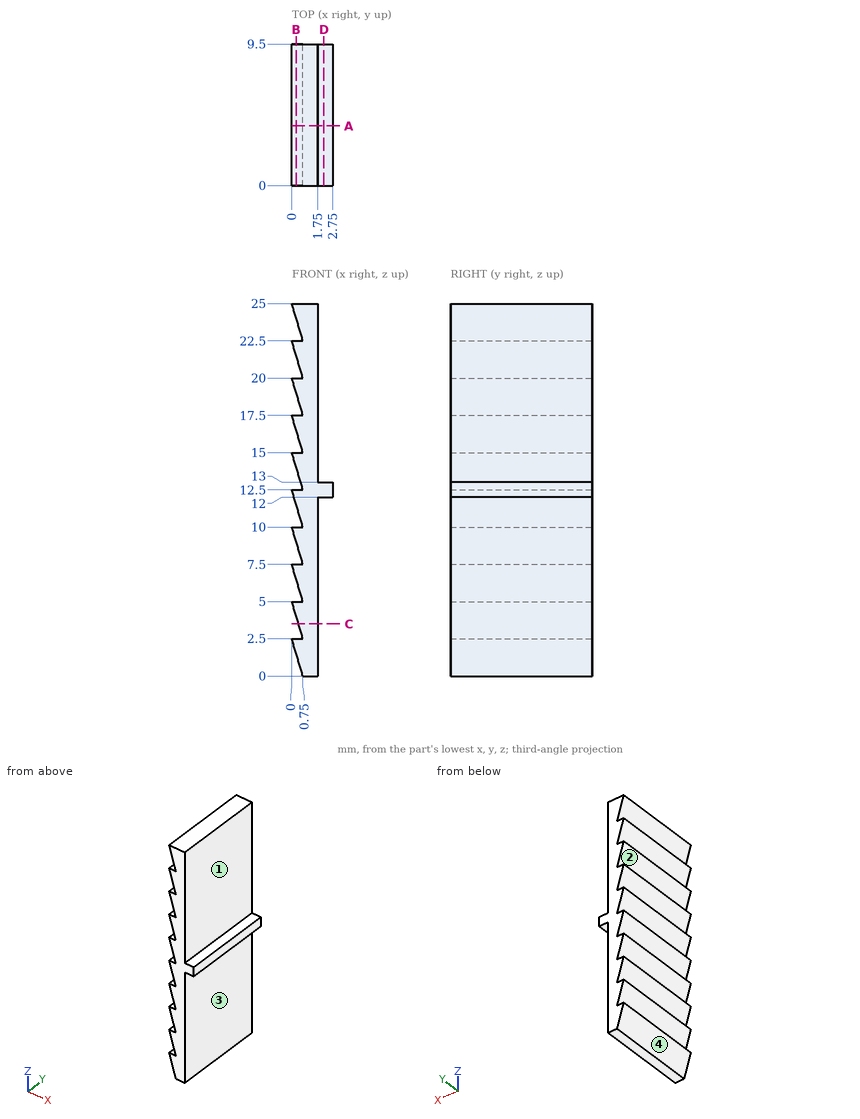
Geometry: see drawing. Coordinates: mm, zero at the bounding-box minimum. A direction names the side the tool comes from. Round coordinates to 2 decimals unless told otherwise and drop trailing zeros. Loops run counter-clockwise (first coordinate to the right, second up) from the corner with the lowest first, then second, coordinate; pieces in that order, holes last. Notation, with made-up numbers: (75, -30.5) -> (131, -30.5) arc R23 cw to (131, -3.5) -> close; hole circle Ø2 at (83, 83). An arc over 180 degrees is marked (long way). One line per question, with ' | ' between items. Start each with the question number.
1. Section B-B on x = 0.3. Count the separate pieces of the cut face and the enclosed holes in it, and give its area (3 significant figures).
2. Section D-D on x = 2.15. Output: boundary loops of the cut face in (y, z).
3. Set-up query: the marked faces 1, 2, 3 and 4. Return all of +Z, -Z, +X, -X, +Y, -Y with unobstructed straight access to the full face (end or side cutting, diameter ignored); none if empty.
4. Line query: line 1 along Z through (x, y) = (2.25, 1.25); line 2 along X through (y, z) = (9, 11.75) (3 decimals); line 3 along X through (y, z) = (0.75, 1.5). Output: solid intervals per line, ascending. Write a range as [from, to].
5. Section C-C on z = 3.5. Output: boundary loops of the cut face in (x, y), and give its area (4 significant figures).
6. Contact query for flat-ended pins moving along their axis: pin 1 (0.8 mm diameter, centred on x = 2.5, y = 2.5, fed in from -Z); pin 2 (3 mm diameter, centred on y = 2.5, z = 7.5, fed in from +X). Output: stop coordinate, or through.
7. Section A-A on y = 4. Output: boundary loops of the cut face in (x, z).
Returned:
1) separate pieces: 10 | enclosed holes: 0 | area: 95.0 mm2
2) outline: (0, 12) -> (9.5, 12) -> (9.5, 13) -> (0, 13) -> close
3) face 1: +Z, +X, +Y, -Y | face 2: -X, +Y, -Y | face 3: -Z, +X, +Y, -Y | face 4: -Z, -X, +Y, -Y
4) line 1: z = [12, 13] | line 2: x = [0.225, 1.75] | line 3: x = [0.3, 1.75]
5) outline: (0.45, 0) -> (1.75, 0) -> (1.75, 9.5) -> (0.45, 9.5) -> close | area: 12.35 mm2
6) pin 1: stops at z = 12 | pin 2: stops at x = 1.75
7) outline: (0, 2.5) -> (0.75, 0) -> (1.75, 0) -> (1.75, 12) -> (2.75, 12) -> (2.75, 13) -> (1.75, 13) -> (1.75, 25) -> (0, 25) -> (0.75, 22.5) -> (0, 22.5) -> (0.75, 20) -> (0, 20) -> (0.75, 17.5) -> (0, 17.5) -> (0.75, 15) -> (0, 15) -> (0.75, 12.5) -> (0, 12.5) -> (0.75, 10) -> (0, 10) -> (0.75, 7.5) -> (0, 7.5) -> (0.75, 5) -> (0, 5) -> (0.75, 2.5) -> close
